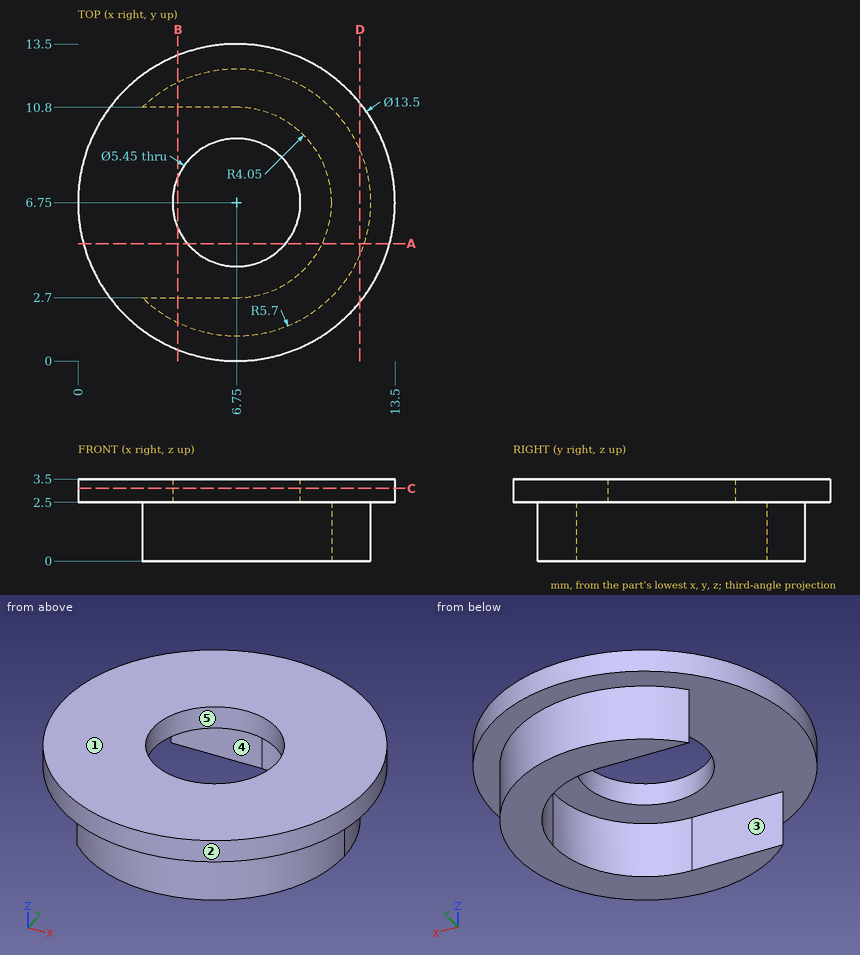
For this review, use the dimensioned drawing (mm, ordinates from the lowest corner) and the shaded views. A direction names the side the tool comes from. Give positions to 0.01 mm unless a question says otherwise; leave off trailing zeros. Order: outer loops, then holes, each group sorted by start corner. A loop starts at its lowest first (then second) coordinate and runs counter-clockwise, first axis right, second up. Notation, with made-up numbers: (51.25, -17.75) - (55.25, -17.75) arc R22 cw to (55.25, 8.25) - close; hole circle Ø3 at (-35.5, -7.75). An arc over 180 degrees is marked (long way). Use CSV: the item, a comma, the result in double quotes. Start each with the question number.
Q1. Take a section at A-A (y = 5). State the section outline as (x, z) points, and give its area (3 significant figures).
Q2. Draft analysis for pull direction Y (two halves, no side actions). For the marked faces 1, 2 and 3, state which applies: pulls with the +Y half, pulls with the -Y half, needs draft (parallel to the pull), parting line crosses it, or undercut.
Q3. Take a section at D-D (x = 12). State the section outline as (y, z) points, and give its area (3 significant figures).
Q4. For line 1 (Y direction, x = 6.75, z = 2.7) (3 decimals); line 2 (Z direction, x = 4.25, y = 3.5); line 3 (Y direction, x = 10.25, z = 1.1), list the stretches that pass through material, from the lowest coordinate up.
Q5. For P1, Ø2, axis at x = 9, y = 6.5, coming from the -Z side; P2, Ø1.2, axis at x = 4.5, z = 0.5, coming from the +Y side; P3, Ø0.8, axis at x = 4.5, z = 1.5, coming from the -Y side, all flat-tipped, find the tip position at first contact; note any pin that passes through.
Q6. Machinability: for the marked faces 4 and 5, which of the approach directions +Z, -Z, +X, -X, +Y, -Y give a long, thin tool a straight path to every point of the face, cutting with its end or side? Answer none if there is none.
Q7. Take a section at C-C (z = 3.1). State the section outline as (x, y) points (3 decimals).
Q8. Take a section at B-B (x = 4.25). State the section outline as (y, z) points, and give its area (3 significant figures).
Calculated:
1,outline,"(0.23, 2.5) - (4.66, 2.5) - (4.66, 3.5) - (0.23, 3.5) - close; (8.84, 2.5) - (10.4, 2.5) - (10.4, 0) - (12.17, 0) - (12.17, 2.5) - (13.27, 2.5) - (13.27, 3.5) - (8.84, 3.5) - close"
1,area,"13.3 mm²"
2,face 1,"needs draft"
2,face 2,"parting line crosses it"
2,face 3,"undercut"
3,outline,"(2.51, 2.5) - (4.53, 2.5) - (4.53, 0) - (8.97, 0) - (8.97, 2.5) - (10.99, 2.5) - (10.99, 3.5) - (2.51, 3.5) - close"
3,area,"19.6 mm²"
4,line 1,"y = 0 to 4.025, 9.475 to 13.5"
4,line 2,"z = 2.5 to 3.5"
4,line 3,"y = 2.25 to 4.71, 8.79 to 11.25"
5,P1,"stops at z = 2.5"
5,P2,"stops at y = 12.21"
5,P3,"stops at y = 1.36"
6,face 4,"-Z, -X"
6,face 5,"+Z, -Z"
7,outline,"circle Ø13.5 at (6.75, 6.75); hole circle Ø5.45 at (6.75, 6.75)"
8,outline,"(0.48, 2.5) - (1.63, 2.5) - (1.63, 0) - (2.7, 0) - (2.7, 2.5) - (5.67, 2.5) - (5.67, 3.5) - (0.48, 3.5) - close; (7.83, 2.5) - (10.8, 2.5) - (10.8, 0) - (11.87, 0) - (11.87, 2.5) - (13.02, 2.5) - (13.02, 3.5) - (7.83, 3.5) - close"
8,area,"15.7 mm²"
